Geometry check sheet. Reference: the model listing, model coordinates, mm. Face numbers are marked on the shaded views. A direction names the side the tool comes from. Round coordinates to 2 decimals unless told otherwise and drop trailing zeros. Order: outer loops, then holes, each group sorted by start corner. A loop starts at its lowest first (then second) coordinate and runs counter-clockwise, first axis right, second up. Notation, with made-up numbers: (25, 16.5) - (35, 16.5) arc R21 cw to (35, 45.5) - close; hole circle Ø1 at (74.25, -20). An arc over 180 degrees is marked (long way). Write each question's results on one line, items separated by ' | '.
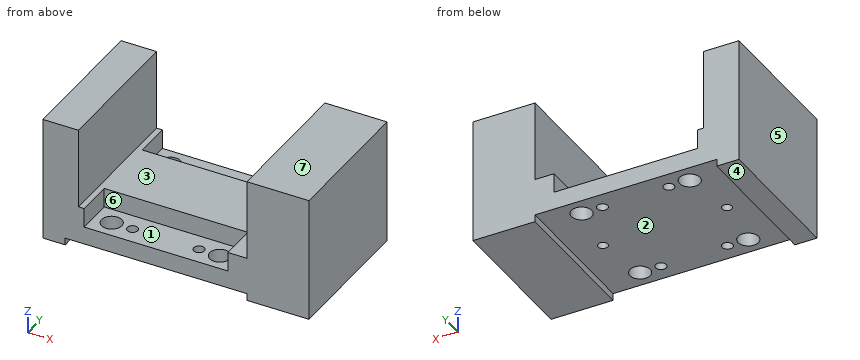
```python
from build123d import *

# Parameters (mm, degrees)
SKETCH_1_W           = 30
SKETCH_1_H           = 28
EXTRUDE_1_DEPTH      = 10
CUT_EXTRUDE_2_DEPTH  = 0.8
M1_4X0_3_2_D         = 1.1
M1_4X0_3_2_DEPTH     = 3.7
M1_4X0_3_2_TIP       = 0.33047334
SKETCH_12_W          = 30
SKETCH_12_H          = 4.25
CUT_EXTRUDE_5_DEPTH  = 10
SKETCH_14_W          = 23
SKETCH_14_H          = 23.75
CUT_EXTRUDE_7_DEPTH  = 5
SKETCH_23_W          = 4
SKETCH_23_H          = 23.75
EXTRUDE_4_DEPTH      = 9.1
SKETCH_31_W          = 7
SKETCH_31_H          = 23.75
EXTRUDE_6_DEPTH      = 4.1
SKETCH_32_W          = 30
SKETCH_32_H          = 7.75
CUT_EXTRUDE_13_DEPTH = 20
SKETCH_33_W          = 3
SKETCH_33_H          = 0.8
CUT_EXTRUDE_14_DEPTH = 10
SKETCH_24_W          = 16.2
SKETCH_24_H          = 4.1
CUT_EXTRUDE_10_DEPTH = 5
SKETCH_29_W          = 16.2
SKETCH_29_H          = 2
EXTRUDE_5_DEPTH      = 4.1
SKETCH_35_W          = 16.2
SKETCH_35_H          = 2
EXTRUDE_7_DEPTH      = 4.1
SKETCH_30_R          = 1.15
SKETCH_30_R_2        = 0.6
CUT_EXTRUDE_12_DEPTH = 5


with BuildPart() as part:
    # 草图1 → 凸台-拉伸1 (new body)
    with BuildSketch(Plane.XY):
        with Locations((7.449728974, 2.736434109)):
            Rectangle(SKETCH_1_W, SKETCH_1_H)
    extrude(amount=EXTRUDE_1_DEPTH)

    # 草图2 → 切除-拉伸2 (cut)
    with BuildSketch(Plane(origin=(0, 0, 0), x_dir=(-1, 0, 0), z_dir=(0, 0, -1))):
        with BuildLine():
            Line((5.050271026, 16.736434109), (-15.449728974, 16.736434109))
            Line((-15.449728974, 16.736434109), (-15.449728974, 3.736434109))
            ThreePointArc((-15.449728974, 3.736434109), (-14.571049317, 1.615113765), (-12.449728974, 0.736434109))
            Line((-12.449728974, 0.736434109), (2.050271026, 0.736434109))
            ThreePointArc((2.050271026, 0.736434109), (4.17159137, 1.615113765), (5.050271026, 3.736434109))
            Line((5.050271026, 3.736434109), (5.050271026, 16.736434109))
        make_face()
    extrude(amount=-CUT_EXTRUDE_2_DEPTH, mode=Mode.SUBTRACT)

    # M1.4x0.3 螺纹孔2
    with Locations(Plane(origin=(0, 0, 0.8), x_dir=(-1, 0, 0), z_dir=(0, 0, -1))):
        with Locations((-12.199728974, 8.736434109), (1.800271026, 8.736434109)):
            Hole(M1_4X0_3_2_D / 2, depth=M1_4X0_3_2_DEPTH)
            with Locations((0, 0, -(M1_4X0_3_2_DEPTH + M1_4X0_3_2_TIP / 2))):  # 118° drill point
                Cone(0, M1_4X0_3_2_D / 2, M1_4X0_3_2_TIP, mode=Mode.SUBTRACT)

    # 草图12 → 切除-拉伸5 (cut)
    with BuildSketch(Plane(origin=(0, 0, 0), x_dir=(-1, 0, 0), z_dir=(0, 0, -1))):
        with Locations((-7.449728974, -9.138565891)):
            Rectangle(SKETCH_12_W, SKETCH_12_H)
    extrude(amount=-CUT_EXTRUDE_5_DEPTH, mode=Mode.SUBTRACT)

    # 草图14 → 切除-拉伸7 (cut)
    with BuildSketch(Plane.XY.offset(10)):
        with Locations((3.949728974, 4.861434109)):
            Rectangle(SKETCH_14_W, SKETCH_14_H)
    extrude(amount=-CUT_EXTRUDE_7_DEPTH, mode=Mode.SUBTRACT)

    # 草图23 → 凸台-拉伸4 (add)
    with BuildSketch(Plane.XY.offset(5)):
        with Locations((-5.550271026, 4.861434109)):
            Rectangle(SKETCH_23_W, SKETCH_23_H)
    extrude(amount=EXTRUDE_4_DEPTH)

    # 草图31 → 凸台-拉伸6 (add)
    with BuildSketch(Plane.XY.offset(10)):
        with Locations((18.949728974, 4.861434109)):
            Rectangle(SKETCH_31_W, SKETCH_31_H)
    extrude(amount=EXTRUDE_6_DEPTH)

    # 草图32 → 切除-拉伸13 (cut)
    with BuildSketch(Plane(origin=(0, 0, 0), x_dir=(-1, 0, 0), z_dir=(0, 0, -1))):
        with Locations((-7.449728974, -3.138565891)):
            Rectangle(SKETCH_32_W, SKETCH_32_H)
    extrude(amount=-CUT_EXTRUDE_13_DEPTH, mode=Mode.SUBTRACT)

    # 草图33 → 切除-拉伸14 (cut)
    with BuildSketch(Plane.XZ.offset(-0.736434109)):
        with Locations((-3.550271026, 0.4)):
            Rectangle(SKETCH_33_W, SKETCH_33_H)
        with Locations((13.949728974, 0.4)):
            Rectangle(SKETCH_33_W, SKETCH_33_H)
    extrude(amount=-CUT_EXTRUDE_14_DEPTH, mode=Mode.SUBTRACT)

    # 草图24 → 切除-拉伸10 (cut)
    with BuildSketch(Plane(origin=(0, 0, 0.8), x_dir=(-1, 0, 0), z_dir=(0, 0, -1))):
        with Locations((-5.199728974, 14.686434109)):
            Rectangle(SKETCH_24_W, SKETCH_24_H)
        with Locations((-5.199728974, 2.786434109)):
            Rectangle(SKETCH_24_W, SKETCH_24_H)
    extrude(amount=-CUT_EXTRUDE_10_DEPTH, mode=Mode.SUBTRACT)

    # 草图29 → 凸台-拉伸5 (add)
    with BuildSketch(Plane(origin=(0, 12.636434109, 0), x_dir=(1, 0, 0), z_dir=(0, 1, 0))):
        with Locations((5.199728974, -1.8)):
            Rectangle(SKETCH_29_W, SKETCH_29_H)
    extrude(amount=EXTRUDE_5_DEPTH)

    # 草图35 → 凸台-拉伸7 (add)
    with BuildSketch(Plane.XZ.offset(-4.836434109)):
        with Locations((5.199728974, 1.8)):
            Rectangle(SKETCH_35_W, SKETCH_35_H)
    extrude(amount=EXTRUDE_7_DEPTH)

    # 草图30 → 切除-拉伸12 (cut)
    with BuildSketch(Plane(origin=(0, 0, 0.8), x_dir=(-1, 0, 0), z_dir=(0, 0, -1))):
        with Locations((0.900271026, 14.736434109)):
            Circle(SKETCH_30_R)
        with Locations((-11.299728974, 14.736434109)):
            Circle(SKETCH_30_R)
        with Locations((-8.949728974, 2.736434109)):
            Circle(SKETCH_30_R_2)
        with Locations((-1.449728974, 14.736434109)):
            Circle(SKETCH_30_R_2)
        with Locations((-8.949728974, 14.736434109)):
            Circle(SKETCH_30_R_2)
        with Locations((-1.449728974, 2.736434109)):
            Circle(SKETCH_30_R_2)
        with Locations((-11.299728974, 2.736434109)):
            Circle(SKETCH_30_R)
        with Locations((0.900271026, 2.736434109)):
            Circle(SKETCH_30_R)
    extrude(amount=-CUT_EXTRUDE_12_DEPTH, mode=Mode.SUBTRACT)


solid = part.part
```
(1) Access from +Z, -Z, +X, -X, +Y, -Y to the whole of each face (thin tool, end or side, straight path). Record for the marked faces 1, 2, 3 and 4.
Answers follow:
face 1: +Z, -Y | face 2: -Z, +Y, -Y | face 3: +Z, +Y, -Y | face 4: -Z, +X, -X, +Y, -Y
(2) Depth check by flat-ended pin: pin 1 Ø2 at (x, y) = (11.3, 14.74) entering from +Z; pin 2 Ø4.5 at (x, y) = (1.5, 14) entering from +Z; pin 3 Ø1.4 at (x, y) = (8.95, 2.74) entering from -Z; pin 4 Ø0.7 at (x, y) = (12.2, 8.74) entering from -Z. Enter the tip coordinate at first touch or a pass-through.
Answers follow:
pin 1: through | pin 2: z = 5 | pin 3: z = 0.8 | pin 4: z = 4.62
(3) Draft check along X on the marked faces 5, 6 and 7. Enter one of: released by +X, released by -X, zero draft, split by the parting line, or undercut.
Answers follow:
face 5: released by -X | face 6: undercut | face 7: zero draft
(4) Material ranges on line 1 (X direction, y = 9.25, z = 6); line 2 (X direction, y = 2.75, z = 3.75); line 3 (Y direction, x = 3.25, z = 3), recorded low to high.
Answers follow:
line 1: -7.55 to -3.55, 15.45 to 22.45 | line 2: -7.55 to -2.9, 13.3 to 22.45 | line 3: 4.84 to 12.64
(5) Section check B-B (x = 3). Record the cut outline in (y, z), then the cut area to 3 significant figures.
Answers follow:
outline: (0.74, 0.8) - (16.74, 0.8) - (16.74, 2.8) - (12.64, 2.8) - (12.64, 5) - (4.84, 5) - (4.84, 2.8) - (0.74, 2.8) - close | area: 49.2 mm²
(6) Section check A-A (z = 6.5). Record the cut outline in (x, y), then the cut area to 3 significant figures.
Answers follow:
outline: (-7.55, 0.74) - (-3.55, 0.74) - (-3.55, 16.74) - (-7.55, 16.74) - close; (15.45, 0.74) - (22.45, 0.74) - (22.45, 16.74) - (15.45, 16.74) - close | area: 176 mm²
(7) Section check D-D (y = 7.75). Record the cut outline in (x, z).
Answers follow:
outline: (-7.55, 0) - (-5.05, 0) - (-5.05, 0.8) - (15.45, 0.8) - (15.45, 0) - (22.45, 0) - (22.45, 14.1) - (15.45, 14.1) - (15.45, 5) - (-3.55, 5) - (-3.55, 14.1) - (-7.55, 14.1) - close
(8) Section check C-C (x = 11). Record the cut outline in (y, z), then the cut area to 3 significant figures.
Answers follow:
outline: (0.74, 0.8) - (1.63, 0.8) - (1.63, 2.8) - (0.74, 2.8) - close; (3.85, 0.8) - (13.63, 0.8) - (13.63, 2.8) - (12.64, 2.8) - (12.64, 5) - (4.84, 5) - (4.84, 2.8) - (3.85, 2.8) - close; (15.85, 0.8) - (16.74, 0.8) - (16.74, 2.8) - (15.85, 2.8) - close | area: 40.3 mm²
